from build123d import *

# Parameters (mm, degrees)
F0_R     = 1.5
F1_DEPTH = 5
F2_W     = 50.6
F2_H     = 86.6
F2_R     = 1.5
F3_DEPTH = 5
F4_R     = 1.1
F5_DEPTH = 5
F7_DEPTH = 2


with BuildPart() as f1:
    # F0 (on Top) → F1 (new body)
    with BuildSketch(Plane.XY):
        with BuildLine():
            Line((-25, -48), (25, -48))
            ThreePointArc((25, -48), (28.535534, -46.535534), (30, -43))
            Line((30, -43), (30, 43))
            ThreePointArc((30, 43), (28.535534, 46.535534), (25, 48))
            Line((25, 48), (-27, 48))
            Line((-27, 48), (-30, 48))
            Line((-30, 48), (-30, 43))
            Line((-30, 43), (-30, -43))
            ThreePointArc((-30, -43), (-28.535534, -46.535534), (-25, -48))
        make_face()
        with Locations((-22, -36.08)):
            Circle(F0_R, mode=Mode.SUBTRACT)
        with Locations((22, -36.08)):
            Circle(F0_R, mode=Mode.SUBTRACT)
        with Locations((-22, 40)):
            Circle(F0_R, mode=Mode.SUBTRACT)
        with Locations((22, 40)):
            Circle(F0_R, mode=Mode.SUBTRACT)
    extrude(amount=F1_DEPTH)

    # F2 (on face) → F3 (cut)
    with BuildSketch(Plane.XY.offset(5)):
        Rectangle(F2_W, F2_H)
        with Locations((-22, -36.08)):
            Circle(F2_R, mode=Mode.SUBTRACT)
        with Locations((22, -36.08)):
            Circle(F2_R, mode=Mode.SUBTRACT)
        with Locations((-22, 40)):
            Circle(F2_R, mode=Mode.SUBTRACT)
        with Locations((22, 40)):
            Circle(F2_R, mode=Mode.SUBTRACT)
    extrude(amount=-F3_DEPTH, mode=Mode.SUBTRACT)

    # F4 (on face) → F5 (join)
    with BuildSketch(Plane.XY.offset(5)):
        with BuildLine():
            Line((-18.3, 43.3), (-25.3, 43.3))
            Line((-25.3, 43.3), (-25.3, 36.9))
            Line((-25.3, 36.9), (-21.3, 36.9))
            ThreePointArc((-21.3, 36.9), (-19.17868, 37.77868), (-18.3, 39.9))
            Line((-18.3, 39.9), (-18.3, 43.3))
        make_face()
        with Locations((-22, 40)):
            Circle(F4_R, mode=Mode.SUBTRACT)
        with BuildLine():
            Line((25.3, 36.9), (25.3, 43.3))
            Line((25.3, 43.3), (18.3, 43.3))
            Line((18.3, 43.3), (18.3, 39.9))
            ThreePointArc((18.3, 39.9), (19.17868, 37.77868), (21.3, 36.9))
            Line((21.3, 36.9), (25.3, 36.9))
        make_face()
        with Locations((22, 40)):
            Circle(F4_R, mode=Mode.SUBTRACT)
        with BuildLine():
            Line((18.3, -43.3), (25.3, -43.3))
            Line((25.3, -43.3), (25.3, -32.9))
            Line((25.3, -32.9), (21.3, -32.9))
            ThreePointArc((21.3, -32.9), (19.17868, -33.77868), (18.3, -35.9))
            Line((18.3, -35.9), (18.3, -43.3))
        make_face()
        with Locations((22, -36.08)):
            Circle(F4_R, mode=Mode.SUBTRACT)
        with BuildLine():
            Line((-25.3, -32.9), (-25.3, -43.3))
            Line((-25.3, -43.3), (-18.3, -43.3))
            Line((-18.3, -43.3), (-18.3, -35.9))
            ThreePointArc((-18.3, -35.9), (-19.17868, -33.77868), (-21.3, -32.9))
            Line((-21.3, -32.9), (-25.3, -32.9))
        make_face()
        with Locations((-22, -36.08)):
            Circle(F4_R, mode=Mode.SUBTRACT)
    extrude(amount=-F5_DEPTH)

    # F6 (on face) → F7 (join)
    with BuildSketch(Plane.XY.offset(5)):
        with BuildLine():
            Line((25, 48), (-30, 48))
            Line((-30, 48), (-30, -43))
            ThreePointArc((-30, -43), (-28.535534, -46.535534), (-25, -48))
            Line((-25, -48), (25, -48))
            ThreePointArc((25, -48), (28.535534, -46.535534), (30, -43))
            Line((30, -43), (30, 43))
            ThreePointArc((30, 43), (28.535534, 46.535534), (25, 48))
        make_face()
        with BuildLine():
            Line((-23, 34.7), (-20, 34.7))
            Line((-20, 34.7), (20, 34.7))
            ThreePointArc((20, 34.7), (22.12132, 33.82132), (23, 31.7))
            Line((23, 31.7), (23, -22.3))
            ThreePointArc((23, -22.3), (22.12132, -24.42132), (20, -25.3))
            Line((20, -25.3), (-20, -25.3))
            ThreePointArc((-20, -25.3), (-22.12132, -24.42132), (-23, -22.3))
            Line((-23, -22.3), (-23, 31.7))
            Line((-23, 31.7), (-23, 34.7))
        make_face(mode=Mode.SUBTRACT)
    extrude(amount=F7_DEPTH)


solid = f1.part
Work out the finished part from the listing and answer in its coordinate system (mm). A direction names the side the tool comes from. Give positions to 0.01 mm unless a question says otherwise; leave off trailing zeros. Loops run counter-clockwise (first coordinate to the right, second up) from the corner with the lowest first, then second, coordinate; pieces in that order, holes last. Notation, with made-up numbers: (69, 24.25) -> (76, 24.25) arc R14 ccw to (76, 44.25) -> close; hole circle Ø9 at (78, -6.5). An arc over 180 degrees is marked (long way). Use a Markdown table: item, result. Add a question column.
1) The part is cut by section B-B, the plane y = 15. Determine the outline of the cut face in (x, z), plus the area to 3 significant figures.
2) For a pull along Y with two mould halves and no side action, classify faces 1 (the flat face through (-23, 36.9, 3)), 2 (the flat face through (-2, 48, 3)), 3 (the flat face through (30, -1, 3)) as +Y half, -Y half, draft (parallel to the pull), parting line (faces both ways), or undercut.
3) The part is cut by section A-A, the plane x = -15.5. Determine the outline of the cut face in (y, z).
4) Which of the six approach directions +Z, -Z, +X, -X, +Y, -Y give full straight-line access (tool end or side, diameter ignored) to faces 4 (the flat face through (-18.3, 42, 3)), 5 (the cylindrical face through (-22.1, -24.44, 5.99)), 6 (the cylindrical face through (28, -47, 3))?
5) Consider line 1 along Y through (x, z) = (22, 3.45); line 2 along X through (y, z) = (-20.5, 2.25); line 3 along Y through (x, z) = (-16.5, 0.75). Determine where each line is inside the solid, lowest interval first.
6) Each of these flat-tipped pins is pushed along its axis until it touches: P1, Ø2.5, axis at x = -22.5, y = 39.5, coming from the -Z side; P2, Ø0.7, axis at x = -22, y = -36, coming from the -Z side. Where does it stop, or does it pass through?
7) The part is cut by section C-C, the plane z = 3.5. Determine the outline of the cut face in (x, y), plus the area to 3 significant figures.
Reported:
| question | item | result |
|---|---|---|
| 1 | outline | (-30, 0) -> (-25.3, 0) -> (-25.3, 5) -> (-23, 5) -> (-23, 7) -> (-30, 7) -> close; (23, 5) -> (25.3, 5) -> (25.3, 0) -> (30, 0) -> (30, 7) -> (23, 7) -> close |
| 1 | area | 75.0 mm^2 |
| 2 | face 1 | undercut |
| 2 | face 2 | +Y half |
| 2 | face 3 | draft |
| 3 | outline | (-48, 0) -> (-43.3, 0) -> (-43.3, 5) -> (-25.3, 5) -> (-25.3, 7) -> (-48, 7) -> close; (34.7, 5) -> (43.3, 5) -> (43.3, 0) -> (48, 0) -> (48, 7) -> (34.7, 7) -> close |
| 4 | face 4 | -Z |
| 4 | face 5 | +Z, -Z |
| 4 | face 6 | +Z, -Z, +X, -Y |
| 5 | line 1 | y = -48 to -37.18, -34.98 to -32.9, 36.9 to 38.9, 41.1 to 48 |
| 5 | line 2 | x = -30 to -25.3, 25.3 to 30 |
| 5 | line 3 | y = -48 to -43.3, 43.3 to 48 |
| 6 | P1 | stops at z = 0 |
| 6 | P2 | stops at z = 5 |
| 7 | outline | (-30, -43) arc R5 ccw to (-25, -48) -> (25, -48) arc R5 ccw to (30, -43) -> (30, 43) arc R5 ccw to (25, 48) -> (-30, 48) -> close; hole (-25.3, -32.9) -> (-21.3, -32.9) arc R3 cw to (-18.3, -35.9) -> (-18.3, -43.3) -> (18.3, -43.3) -> (18.3, -35.9) arc R3 cw to (21.3, -32.9) -> (25.3, -32.9) -> (25.3, 36.9) -> (21.3, 36.9) arc R3 cw to (18.3, 39.9) -> (18.3, 43.3) -> (-18.3, 43.3) -> (-18.3, 39.9) arc R3 cw to (-21.3, 36.9) -> (-25.3, 36.9) -> close; hole circle Ø2.2 at (-22, -36.08); hole circle Ø2.2 at (-22, 40); hole circle Ø2.2 at (22, -36.08); hole circle Ø2.2 at (22, 40) |
| 7 | area | 1,570 mm^2 |
